from build123d import *

# Parameters (mm, degrees)
BEARING_MOUNT_BLOCK_DEPTH                      = 10.16
BEARING_MOUNT_BLOCK_DEPTH_BACK                 = 5.08
SKETCH1_W                                      = 36.576
SKETCH1_H                                      = 33.274
ENCODER_EXTENSION_DEPTH                        = 14.5034
ENCODER_MOUNT_PLATE_DEPTH                      = 6.35
SHAFT_CLEARANCE_HOLE_REACH                     = 56.937
SKETCH6_R                                      = 3.81
F_3_48_TAPPED_HOLES_D                          = 1.9939
CBORE_FOR_4_SOCKET_HEAD_CAP_SCREW1_D           = 3.2639
CBORE_FOR_4_SOCKET_HEAD_CAP_SCREW1_DEPTH       = 12.7
CBORE_FOR_4_SOCKET_HEAD_CAP_SCREW1_CBORE_D     = 4.09575
CBORE_FOR_4_SOCKET_HEAD_CAP_SCREW1_CBORE_DEPTH = 4.7625
CBORE_FOR_4_SOCKET_HEAD_CAP_SCREW1_TIP         = 0.980574487
CBORE_FOR_4_SOCKET_HEAD_CAP_SCREW2_D           = 3.2639
CBORE_FOR_4_SOCKET_HEAD_CAP_SCREW2_DEPTH       = 12.7
CBORE_FOR_4_SOCKET_HEAD_CAP_SCREW2_CBORE_D     = 4.09575
CBORE_FOR_4_SOCKET_HEAD_CAP_SCREW2_CBORE_DEPTH = 4.7625
CBORE_FOR_4_SOCKET_HEAD_CAP_SCREW2_TIP         = 0.980574487
MATERIAL_REDUCTION_CHAMFER_SIZE                = 10.16
CHAMFER1_SIZE                                  = 0.508


with BuildPart() as part:
    # Sketch1 → Bearing Mount Block (new, two sides: drawn at the far end of the back side and taken through both)
    with BuildSketch(Plane.XY.offset(-BEARING_MOUNT_BLOCK_DEPTH_BACK)):
        Rectangle(SKETCH1_W, SKETCH1_H)
    extrude(amount=BEARING_MOUNT_BLOCK_DEPTH + BEARING_MOUNT_BLOCK_DEPTH_BACK)

    # Sketch3 → Encoder Extension (add)
    with BuildSketch(Plane(origin=(0, 0, -5.08), x_dir=(-1, 0, 0), z_dir=(0, 0, -1))):
        with BuildLine():
            Line((18.288, 16.637), (-18.288, 16.637))
            Line((-18.288, 16.637), (-18.288, -16.637))
            Line((-18.288, -16.637), (-8.22643419, -16.637))
            ThreePointArc((-8.22643419, -16.637), (0, -13.5763), (8.22643419, -16.637))
            Line((8.22643419, -16.637), (18.288, -16.637))
            Line((18.288, -16.637), (18.288, 16.637))
        make_face()
    extrude(amount=ENCODER_EXTENSION_DEPTH)

    # Sketch4 → Encoder Mount Plate (add)
    with BuildSketch(Plane(origin=(0, 0, -19.5834), x_dir=(-1, 0, 0), z_dir=(0, 0, -1))):
        with BuildLine():
            Line((18.288, 16.637), (-18.288, 16.637))
            Line((-18.288, 16.637), (-18.288, -16.637))
            Line((-18.288, -16.637), (-9.500261866, -31.703247849))
            ThreePointArc((-9.500261866, -31.703247849), (0, -37.1602), (9.500261866, -31.703247849))
            Line((9.500261866, -31.703247849), (18.288, -16.637))
            Line((18.288, -16.637), (18.288, 16.637))
        make_face()
    extrude(amount=ENCODER_MOUNT_PLATE_DEPTH)

    # Sketch6 → Shaft Clearance Hole (cut, up to next)
    with BuildSketch(Plane(origin=(0, 0, -25.9334), x_dir=(-1, 0, 0), z_dir=(0, 0, -1)), mode=Mode.PRIVATE) as shaft_clearance_hole_sk1:
        with Locations((0, -26.162)):
            Circle(SKETCH6_R)
    shaft_clearance_hole_tool1 = extrude(shaft_clearance_hole_sk1.sketch, amount=-SHAFT_CLEARANCE_HOLE_REACH, mode=Mode.PRIVATE) & part.part
    add(shaft_clearance_hole_tool1.solids().sort_by_distance((0, -26.162, -25.9334))[0], mode=Mode.SUBTRACT)

    # #3-48 Tapped Holes (through all)
    with Locations(Plane(origin=(-3.7211, -19.71686574, -25.9334), x_dir=(-1, 0, 0), z_dir=(0, 0, -1))):
        with Locations((0, 0), (-7.4422, -12.89026852)):
            Hole(F_3_48_TAPPED_HOLES_D / 2)

    # CBORE for #4 Socket Head Cap Screw1
    with Locations(Plane(origin=(-14.2875, -16.637, -2.54), x_dir=(0, 0, -1), z_dir=(0, -1, 0))):
        with Locations((0, 0), (0, 28.575)):
            CounterBoreHole(CBORE_FOR_4_SOCKET_HEAD_CAP_SCREW1_D / 2, CBORE_FOR_4_SOCKET_HEAD_CAP_SCREW1_CBORE_D / 2, CBORE_FOR_4_SOCKET_HEAD_CAP_SCREW1_CBORE_DEPTH, depth=CBORE_FOR_4_SOCKET_HEAD_CAP_SCREW1_DEPTH)
            with Locations((0, 0, -(CBORE_FOR_4_SOCKET_HEAD_CAP_SCREW1_DEPTH + CBORE_FOR_4_SOCKET_HEAD_CAP_SCREW1_TIP / 2))):  # 118° drill point
                Cone(0, CBORE_FOR_4_SOCKET_HEAD_CAP_SCREW1_D / 2, CBORE_FOR_4_SOCKET_HEAD_CAP_SCREW1_TIP, mode=Mode.SUBTRACT)

    # CBORE for #4 Socket Head Cap Screw2
    with Locations(Plane(origin=(0, 16.637, 0), x_dir=(1, 0, 0), z_dir=(0, 1, 0))):
        with Locations((-13.5255, 21.1709), (13.5255, 21.1709), (13.5255, -5.3975), (-13.5255, -5.3975)):
            CounterBoreHole(CBORE_FOR_4_SOCKET_HEAD_CAP_SCREW2_D / 2, CBORE_FOR_4_SOCKET_HEAD_CAP_SCREW2_CBORE_D / 2, CBORE_FOR_4_SOCKET_HEAD_CAP_SCREW2_CBORE_DEPTH, depth=CBORE_FOR_4_SOCKET_HEAD_CAP_SCREW2_DEPTH)
            with Locations((0, 0, -(CBORE_FOR_4_SOCKET_HEAD_CAP_SCREW2_DEPTH + CBORE_FOR_4_SOCKET_HEAD_CAP_SCREW2_TIP / 2))):  # 118° drill point
                Cone(0, CBORE_FOR_4_SOCKET_HEAD_CAP_SCREW2_D / 2, CBORE_FOR_4_SOCKET_HEAD_CAP_SCREW2_TIP, mode=Mode.SUBTRACT)

    # Material Reduction Chamfer
    material_reduction_chamfer_edges = [part.edges().sort_by_distance(p)[0] for p in [
        (0, -16.637, 10.16),
    ]]
    chamfer(material_reduction_chamfer_edges, length=MATERIAL_REDUCTION_CHAMFER_SIZE)

    # Chamfer1
    # the kernel refuses this chamfer: 0.508 mm, written as the material it takes off along each edge
    with BuildSketch(Plane(origin=(13.5255, 16.637, -21.1709), x_dir=(1, 0, 0), z_dir=(0, 0, 1))) as chamfer1_piece_1:
        Polygon((2.047875 + CHAMFER1_SIZE, 0), (2.047875, -CHAMFER1_SIZE), (2.047875, 0), align=None)
    revolve(axis=Axis((13.5255, 16.637, -21.1709), (0, 1, 0)), mode=Mode.SUBTRACT)
    with BuildSketch(Plane(origin=(-13.5255, 16.637, -21.1709), x_dir=(1, 0, 0), z_dir=(0, 0, 1))) as chamfer1_piece_2:
        Polygon((2.047875 + CHAMFER1_SIZE, 0), (2.047875, -CHAMFER1_SIZE), (2.047875, 0), align=None)
    revolve(axis=Axis((-13.5255, 16.637, -21.1709), (0, 1, 0)), mode=Mode.SUBTRACT)
    with BuildSketch(Plane(origin=(3.7211, -32.60713426, -19.5834), x_dir=(1, 0, 0), z_dir=(0, -1, 0))) as chamfer1_piece_3:
        Polygon((0.99695 + CHAMFER1_SIZE, 0), (0.99695, -CHAMFER1_SIZE), (0.99695, 0), align=None)
    revolve(axis=Axis((3.7211, -32.60713426, -19.5834), (0, 0, 1)), mode=Mode.SUBTRACT)
    with BuildSketch(Plane(origin=(-3.7211, -19.71686574, -19.5834), x_dir=(1, 0, 0), z_dir=(0, -1, 0))) as chamfer1_piece_4:
        Polygon((0.99695 + CHAMFER1_SIZE, 0), (0.99695, -CHAMFER1_SIZE), (0.99695, 0), align=None)
    revolve(axis=Axis((-3.7211, -19.71686574, -19.5834), (0, 0, 1)), mode=Mode.SUBTRACT)
    with BuildSketch(Plane(origin=(14.2875, -16.637, -2.54), x_dir=(0, 0, -1), z_dir=(-1, 0, 0))) as chamfer1_piece_5:
        Polygon((2.047875 + CHAMFER1_SIZE, 0), (2.047875, -CHAMFER1_SIZE), (2.047875, 0), align=None)
    revolve(axis=Axis((14.2875, -16.637, -2.54), (0, -1, 0)), mode=Mode.SUBTRACT)
    with BuildSketch(Plane(origin=(-14.2875, -16.637, -2.54), x_dir=(0, 0, -1), z_dir=(-1, 0, 0))) as chamfer1_piece_6:
        Polygon((2.047875 + CHAMFER1_SIZE, 0), (2.047875, -CHAMFER1_SIZE), (2.047875, 0), align=None)
    revolve(axis=Axis((-14.2875, -16.637, -2.54), (0, -1, 0)), mode=Mode.SUBTRACT)
    with BuildSketch(Plane(origin=(-13.5255, 16.637, 5.3975), x_dir=(1, 0, 0), z_dir=(0, 0, 1))) as chamfer1_piece_7:
        Polygon((2.047875 + CHAMFER1_SIZE, 0), (2.047875, -CHAMFER1_SIZE), (2.047875, 0), align=None)
    revolve(axis=Axis((-13.5255, 16.637, 5.3975), (0, 1, 0)), mode=Mode.SUBTRACT)
    with BuildSketch(Plane(origin=(13.5255, 16.637, 5.3975), x_dir=(1, 0, 0), z_dir=(0, 0, 1))) as chamfer1_piece_8:
        Polygon((2.047875 + CHAMFER1_SIZE, 0), (2.047875, -CHAMFER1_SIZE), (2.047875, 0), align=None)
    revolve(axis=Axis((13.5255, 16.637, 5.3975), (0, 1, 0)), mode=Mode.SUBTRACT)


solid = part.part
Input: part model. Units: mm. Frame: model coordinates. A direction names the side the tool comes from. Give positions to 0.01 mm unless a question says otherwise; leave off trailing zeros. Order: outer loops, then holes, each group sorted by start corner. A loop starts at its lowest first (then second) coordinate and runs counter-clockwise, first axis right, second up. Notation, with made-up numbers: (-11, 40.5) - (40, 40.5) arc R25 cw to (40, 75.5) - close; hole circle Ø8 at (72.25, -7.5). An arc over 180 degrees is marked (long way). Answer as a JSON object with one key per item and string values. Group by question number.
Q1. Set-up query: faces 5 (the face through (-15.033, 7.85, 6.023)), 6 (the face through (13.96, -24.06, -22.71)), 7 (the face through (12.694, -7.85, -2.894)). Return all of +Z, -Z, +X, -X, +Y, -Y with unobstructed straight access to the full face (end or side cutting, diameter ignored); none if empty.
Q2. Line query: probe 1 along Z at (x, y) = (6, -15.5); probe 2 along Z at (x, y) = (0, -20.5); probe 3 along Y at (x, z) = (11, -14.5). Output: solid intervals per line, ascending.
Q3. Mould query, pull axis Y, two halves, no side actions, for faces 1 (the face through (11.9, 14.032, -19.925)), 2 (the face through (-3.94, -20.69, -22.97)), 3 (the face through (0.126, -13.577, -12.23)), 4 (the face through (-13.809, 3.127, 5.385)). Classes: pulls with the +Y half, pulls with the -Y half, needs draft (parallel to the pull), parting line crosses it, or undercut.
Q4. Cut plane C-C, the plane x = -6. Output: boundary loops of the cut face in (y, z).
Q5. Cut plane A-A, the plane x = 0. Output: boundary loops of the cut face in (y, z).
Q6. Cut plane D-D, the plane x = 7. Output: boundary loops of the cut face in (y, z).
Q7. Cut plane B-B, the plane z = -8.5. Output: boundary loops of the cut face in (x, y), then the cut area to 3 significant figures.
Q8. First-contact query: pin 1 Ø2 at (x, z) = (-13.53, 5.4) entering from -Y; pin 2 Ø5.5 at (x, z) = (-13.53, 5.4) entering from -Y; pin 3 Ø2.5 at (x, z) = (13.53, -21.17) entering from -Y. Flat tips, straight axial feed; report the tip coordinate or a pass-through.
Results:
{
 "1": {"face 5": "+Y", "face 6": "+Z, -Z, +X, -Y", "face 7": "-Y"},
 "2": {"probe 1": "-25.93 to -19.58, -5.08 to 1.14", "probe 2": "-25.93 to -19.58", "probe 3": "-16.64 to 16.64"},
 "3": {"face 1": "needs draft", "face 2": "undercut", "face 3": "pulls with the -Y half", "face 4": "pulls with the +Y half"},
 "4": {"outline": "(-35.38, -25.93) - (16.64, -25.93) - (16.64, 10.16) - (-6.48, 10.16) - (-16.64, 0) - (-16.64, -5.08) - (-15.1, -5.08) - (-15.1, -19.58) - (-35.38, -19.58) - close"},
 "5": {"outline": "(-37.16, -25.93) - (-29.97, -25.93) - (-29.97, -19.58) - (-37.16, -19.58) - close; (-22.35, -25.93) - (16.64, -25.93) - (16.64, 10.16) - (-6.48, 10.16) - (-16.64, 0) - (-16.64, -5.08) - (-13.58, -5.08) - (-13.58, -19.58) - (-22.35, -19.58) - close"},
 "6": {"outline": "(-34.64, -25.93) - (16.64, -25.93) - (16.64, 10.16) - (-6.48, 10.16) - (-16.64, 0) - (-16.64, -5.08) - (-15.7, -5.08) - (-15.7, -19.58) - (-34.64, -19.58) - close"},
 "7": {"outline": "(-18.29, -16.64) - (-8.23, -16.64) arc R12.59 cw to (8.23, -16.64) - (18.29, -16.64) - (18.29, 16.64) - (-18.29, 16.64) - close", "area": "1,180 mm^2"},
 "8": {"pin 1": "y = -12.24", "pin 2": "y = -13.99", "pin 3": "y = -26.94"}
}
